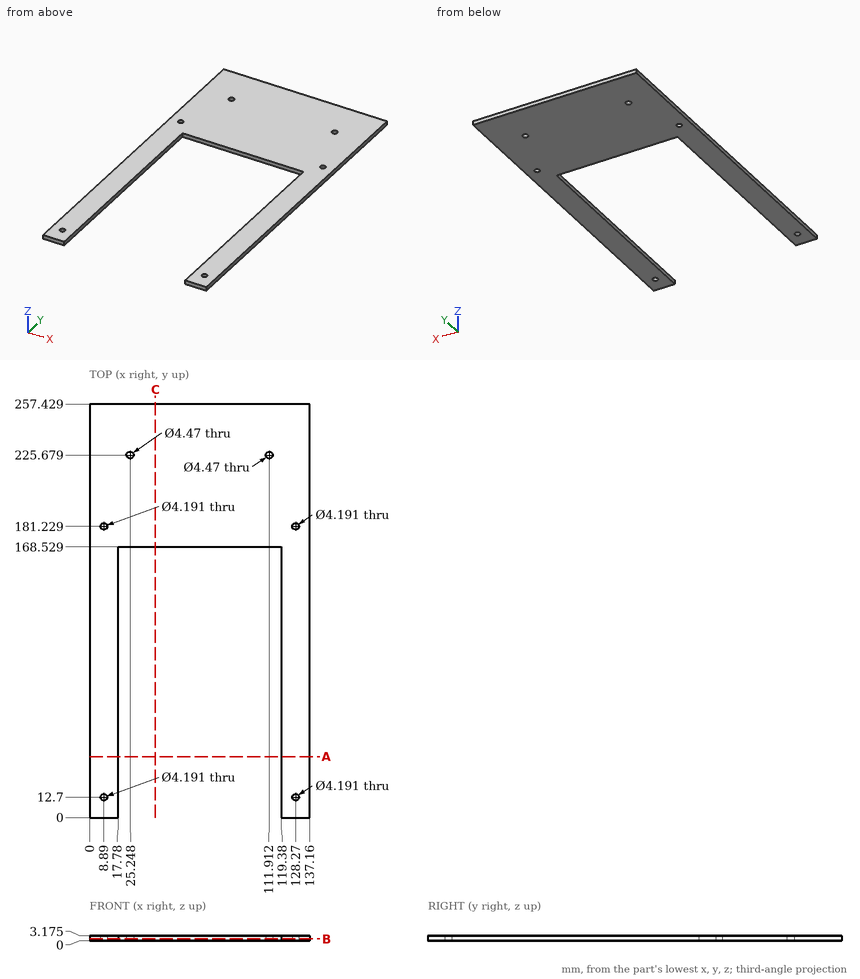
Here's the drawing with two shaded views (mm, measured from the low corner). I have some questions. Give positions to 0.01 mm unless a question says otherwise; leave off trailing zeros. Write each loop counter-clockwise with the first axis right and the second up, starting at its lowest first coordinate (ties: lowest second). Pieces come first, ordered by that corner, then holes. Notation, with made-up numbers: (79.5, -4) -> (90.5, -4) arc R19 cw to (90.5, 32) -> close; hole circle Ø8 at (12, 35). An arc over 180 degrees is marked (long way). Answer as a JSON object with one key per item and string values. Group by question number.
Item 1: I'm going to push a flat-ended pin straight in: P1, Ø3.5, axis at x = 128.27, y = 12.7, coming from the +Z side. Where does the tip first touch, or does it pass through?
Item 2: Suppose I cut it at C-C (x = 41). Please give me the cut outline in (y, z) (1 decimal), plus the area to 3 significant figures.
Item 3: Please list where these lines run through material, in increasing order: line 1 (Y direction, x = 128.27, z = 2.15) (1 decimal); line 2 (X direction, y = 12.7, z = 2.3) (1 decimal); line 3 (X direction, y = 45, z = 1.15). Write a range as [from, to].
Item 4: Suppose I cut it at A-A (y = 38). Please give me the cut outline in (x, z) (1 decimal), plus the area to 3 significant figures.
Item 5: Suppose I cut it at B-B (z = 1.1). Please give me the cut outline in (x, y) (1 decimal), plus the area to 3 significant figures.
Findings:
{
 "1": {"P1": "passes through"},
 "2": {"outline": "(168.5, 0) -> (257.4, 0) -> (257.4, 3.2) -> (168.5, 3.2) -> close", "area": "282 mm²"},
 "3": {"line 1": "y = [0, 10.6], [14.8, 179.1], [183.3, 257.4]", "line 2": "x = [0, 6.8], [11, 17.8], [119.4, 126.2], [130.4, 137.2]", "line 3": "x = [0, 17.78], [119.38, 137.16]"},
 "4": {"outline": "(0, 0) -> (17.8, 0) -> (17.8, 3.2) -> (0, 3.2) -> close; (119.4, 0) -> (137.2, 0) -> (137.2, 3.2) -> (119.4, 3.2) -> close", "area": "113 mm²"},
 "5": {"outline": "(0, 0) -> (17.8, 0) -> (17.8, 168.5) -> (119.4, 168.5) -> (119.4, 0) -> (137.2, 0) -> (137.2, 257.4) -> (0, 257.4) -> close; hole circle Ø4.2 at (8.9, 12.7); hole circle Ø4.2 at (8.9, 181.2); hole circle Ø4.5 at (25.2, 225.7); hole circle Ø4.5 at (111.9, 225.7); hole circle Ø4.2 at (128.3, 12.7); hole circle Ø4.2 at (128.3, 181.2)", "area": "18,100 mm²"}
}
